The model under review builds one solid part; all positions refer to its coordinate system, in mm. Coordinates: 2 decimals unless noted, no trailing zeros. Loops run counter-clockwise (first coordinate to the right, second up) from the corner with the lowest first, then second, coordinate; pieces in that order, holes last. Notation, with made-up numbers: (52, 27) - (64, 27) arc R18 cw to (64, 42) - close; hole circle Ø3 at (63, -27). An arc over 180 degrees is marked (long way). Use a Markdown table: item, result. Add a question column.
1) To check wall thickness, follow L1, parallel to Y at x = 46.5, z = 0.95; L2, parallel to X at y = 17.5, z = 0.35; L3, parallel to X at y = 60.5, z = 0.8. State the ranges of each line that lie inside material, in increasing order. Write a range as [from, to].
2) Add section C-C, the plane z = 0.7. Give the number of separate pieces and of enclosed holes in the cut face, and give its area (3 significant figures).
3) Add section D-D, the plane x = 59.5. Give the boundary of the cut face in (y, z), and give its area (3 significant figures).
4) Add section B-B, the plane x = 45. Give the boundary of the cut face in (y, z), and give its area (3 significant figures).
5) Add section A-A, the plane y = 68. Give the boundary of the cut face in (x, z), and give its area (3 significant figures).
```python
from build123d import *

# Parameters (mm, degrees)
F0_W     = 110
F0_H     = 91
F1_DEPTH = 1
F2_W     = 72
F2_H     = 40
F3_DEPTH = 1.001
F4_R     = 5
F6_DEPTH = 1.001


with BuildPart() as f1:
    # F0 (on Top) → F1 (new body)
    with BuildSketch(Plane.XY):
        with Locations((55, 45.5)):
            Rectangle(F0_W, F0_H)
    extrude(amount=F1_DEPTH)

    # F2 (on face) → F3 (cut, through all)
    with BuildSketch(Plane.XY.offset(1)):
        with Locations((55, 59.718266)):
            Rectangle(F2_W, F2_H)
    extrude(amount=-F3_DEPTH, mode=Mode.SUBTRACT)

    # F4
    f4_edges = [f1.edges().sort_by_distance(p)[0] for p in [
        (0, 91, 0.5),
        (0, 0, 0.5),
        (110, 91, 0.5),
        (110, 0, 0.5),
    ]]
    fillet(f4_edges, radius=F4_R)

    # F5 (on face) → F6 (cut, through all)
    with BuildSketch(Plane.XY.offset(1)):
        with BuildLine():
            Line((30, 27.418266), (23, 27.418266))
            ThreePointArc((23, 27.418266), (20.737258, 26.481008), (19.8, 24.218266))
            Line((19.8, 24.218266), (19.8, 17.218266))
            ThreePointArc((19.8, 17.218266), (20.737258, 14.955525), (23, 14.018266))
            Line((23, 14.018266), (30, 14.018266))
            ThreePointArc((30, 14.018266), (32.262742, 14.955525), (33.2, 17.218266))
            Line((33.2, 17.218266), (33.2, 24.218266))
            ThreePointArc((33.2, 24.218266), (32.262742, 26.481008), (30, 27.418266))
        make_face()
        with BuildLine():
            Line((49, 27.418266), (42, 27.418266))
            ThreePointArc((42, 27.418266), (39.737258, 26.481008), (38.8, 24.218266))
            Line((38.8, 24.218266), (38.8, 17.218266))
            ThreePointArc((38.8, 17.218266), (39.737258, 14.955525), (42, 14.018266))
            Line((42, 14.018266), (49, 14.018266))
            ThreePointArc((49, 14.018266), (51.262742, 14.955525), (52.2, 17.218266))
            Line((52.2, 17.218266), (52.2, 24.218266))
            ThreePointArc((52.2, 24.218266), (51.262742, 26.481008), (49, 27.418266))
        make_face()
        with BuildLine():
            Line((68, 27.418266), (61, 27.418266))
            ThreePointArc((61, 27.418266), (58.737258, 26.481008), (57.8, 24.218266))
            Line((57.8, 24.218266), (57.8, 17.218266))
            ThreePointArc((57.8, 17.218266), (58.737258, 14.955525), (61, 14.018266))
            Line((61, 14.018266), (68, 14.018266))
            ThreePointArc((68, 14.018266), (70.262742, 14.955525), (71.2, 17.218266))
            Line((71.2, 17.218266), (71.2, 24.218266))
            ThreePointArc((71.2, 24.218266), (70.262742, 26.481008), (68, 27.418266))
        make_face()
        with BuildLine():
            Line((87, 27.418266), (80, 27.418266))
            ThreePointArc((80, 27.418266), (77.737258, 26.481008), (76.8, 24.218266))
            Line((76.8, 24.218266), (76.8, 17.218266))
            ThreePointArc((76.8, 17.218266), (77.737258, 14.955525), (80, 14.018266))
            Line((80, 14.018266), (87, 14.018266))
            ThreePointArc((87, 14.018266), (89.262742, 14.955525), (90.2, 17.218266))
            Line((90.2, 17.218266), (90.2, 24.218266))
            ThreePointArc((90.2, 24.218266), (89.262742, 26.481008), (87, 27.418266))
        make_face()
    extrude(amount=-F6_DEPTH, mode=Mode.SUBTRACT)


solid = f1.part
```
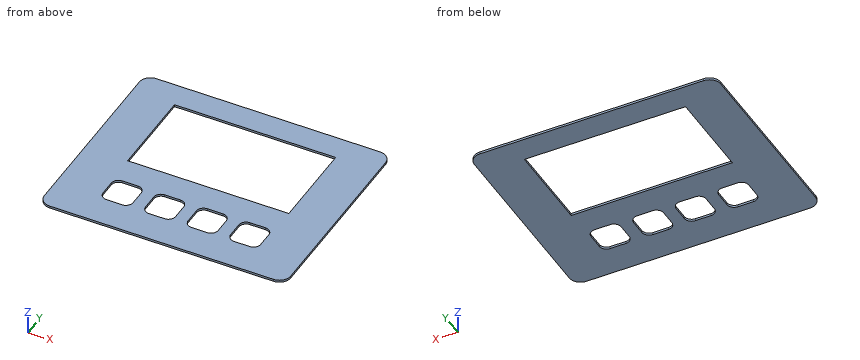
From the geometry:
| question | item | result |
|---|---|---|
| 1 | L1 | y = [0, 14.02], [27.42, 39.72], [79.72, 91] |
| 1 | L2 | x = [0, 19.8], [33.2, 38.8], [52.2, 57.8], [71.2, 76.8], [90.2, 110] |
| 1 | L3 | x = [0, 19], [91, 110] |
| 2 | separate pieces | 1 |
| 2 | enclosed holes | 5 |
| 2 | area | 6,430 mm^2 |
| 3 | outline | (0, 0) - (14.39, 0) - (14.39, 1) - (0, 1) - close; (27.04, 0) - (39.72, 0) - (39.72, 1) - (27.04, 1) - close; (79.72, 0) - (91, 0) - (91, 1) - (79.72, 1) - close |
| 3 | area | 38.3 mm^2 |
| 4 | outline | (0, 0) - (14.02, 0) - (14.02, 1) - (0, 1) - close; (27.42, 0) - (39.72, 0) - (39.72, 1) - (27.42, 1) - close; (79.72, 0) - (91, 0) - (91, 1) - (79.72, 1) - close |
| 4 | area | 37.6 mm^2 |
| 5 | outline | (0, 0) - (19, 0) - (19, 1) - (0, 1) - close; (91, 0) - (110, 0) - (110, 1) - (91, 1) - close |
| 5 | area | 38.0 mm^2 |
